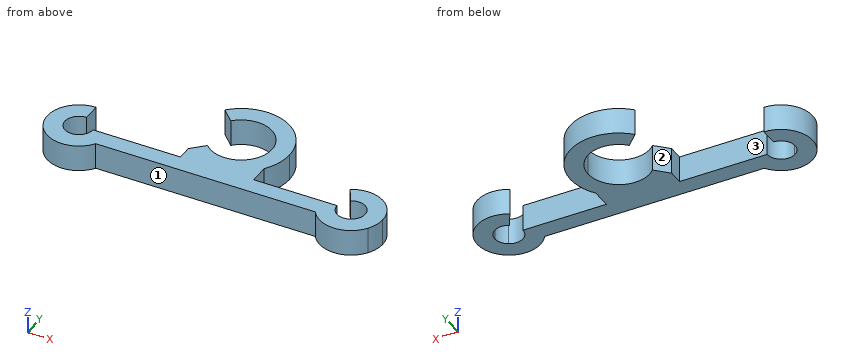
from build123d import *

# Parameters (mm, degrees)
F1_DEPTH = 3


with BuildPart() as f1:
    # F0 (on Top) → F1 (new body)
    with BuildSketch(Plane.XY):
        with BuildLine():
            Line((4.3997598665, -5.5), (0, -5.5))
            Line((0, -5.5), (-3.9389383459, -5.5))
            Line((-3.9389383459, -5.5), (-11.8838464236, -5.5))
            ThreePointArc((-11.8838464236, -5.5), (-12.0388519916, -6.5449944321), (-12.4905205142, -7.5))
            Line((-12.4905205142, -7.5), (12.4905205142, -7.5))
            ThreePointArc((12.4905205142, -7.5), (12.0388519916, -6.5449944321), (11.8838464236, -5.5))
            Line((11.8838464236, -5.5), (4.3997598665, -5.5))
        make_face()
        with BuildLine():
            ThreePointArc((-12.4905205142, -7.5), (-12.0388519916, -6.5449944321), (-11.8838464236, -5.5))
            Line((-11.8838464236, -5.5), (-13.8838464236, -5.5))
            ThreePointArc((-13.8838464236, -5.5), (-14.6838464236, -6.8856406461), (-16.2838464236, -6.8856406461))
            Line((-16.2838464236, -6.8856406461), (-16.638546962, -7.5))
            Line((-16.638546962, -7.5), (-12.4905205142, -7.5))
        make_face()
        with BuildLine():
            Line((-16.638546962, -7.5), (-16.2838464236, -6.8856406461))
            ThreePointArc((-16.2838464236, -6.8856406461), (-17.0293277457, -5.0858895278), (-15.4838464236, -3.9))
            Line((-15.4838464236, -3.9), (-15.4838464236, -1.9))
            ThreePointArc((-15.4838464236, -1.9), (-18.6587479969, -3.8029437252), (-18.4771723331, -7.5))
            Line((-18.4771723331, -7.5), (-16.638546962, -7.5))
        make_face()
        with BuildLine():
            Line((13.8838464236, -5.5), (11.8838464236, -5.5))
            ThreePointArc((11.8838464236, -5.5), (12.0388519916, -6.5449944321), (12.4905205142, -7.5))
            Line((12.4905205142, -7.5), (16.638546962, -7.5))
            Line((16.638546962, -7.5), (16.2838464236, -6.8856406461))
            ThreePointArc((16.2838464236, -6.8856406461), (14.6838464236, -6.8856406461), (13.8838464236, -5.5))
        make_face()
        with BuildLine():
            ThreePointArc((19.0838464236, -5.5), (17.2838464236, -2.3823085464), (13.6838464236, -2.3823085464))
            Line((13.6838464236, -2.3823085464), (14.6838464236, -4.1143593539))
            ThreePointArc((14.6838464236, -4.1143593539), (16.2838464236, -4.1143593539), (17.0838464236, -5.5))
            ThreePointArc((17.0838464236, -5.5), (16.8694870697, -6.3), (16.2838464236, -6.8856406461))
            Line((16.2838464236, -6.8856406461), (16.638546962, -7.5))
            Line((16.638546962, -7.5), (18.4771723331, -7.5))
            ThreePointArc((18.4771723331, -7.5), (18.9288408557, -6.5449944321), (19.0838464236, -5.5))
        make_face()
        with BuildLine():
            ThreePointArc((-2.5065971292, 2.4427383879), (1.3185048441, 3.2421512883), (3.5, 0))
            ThreePointArc((3.5, 0), (1.3185048441, -3.2421512883), (-2.5065971292, -2.4427383879))
            Line((-2.5065971292, -2.4427383879), (-3.9389383459, -3.8385888953))
            ThreePointArc((-3.9389383459, -3.8385888953), (-2.1374939855, -5.0676542366), (0, -5.5))
            ThreePointArc((0, -5.5), (2.4594957974, -4.9194390354), (4.3997598665, -3.3003201537))
            ThreePointArc((4.3997598665, -3.3003201537), (5.2176948582, -1.7394425449), (5.5, 0))
            ThreePointArc((5.5, 0), (2.0719361836, 5.0948091673), (-3.9389383459, 3.8385888953))
            Line((-3.9389383459, 3.8385888953), (-2.5065971292, 2.4427383879))
        make_face()
        with BuildLine():
            ThreePointArc((0, -5.5), (-2.1374939855, -5.0676542366), (-3.9389383459, -3.8385888953))
            Line((-3.9389383459, -3.8385888953), (-3.9389383459, -5.5))
            Line((-3.9389383459, -5.5), (0, -5.5))
        make_face()
        with BuildLine():
            ThreePointArc((4.3997598665, -3.3003201537), (2.4594957974, -4.9194390354), (0, -5.5))
            Line((0, -5.5), (4.3997598665, -5.5))
            Line((4.3997598665, -5.5), (4.3997598665, -3.3003201537))
        make_face()
        with BuildLine():
            Line((16.638546962, -7.5), (12.4905205142, -7.5))
            ThreePointArc((12.4905205142, -7.5), (15.4838464236, -9.1), (18.4771723331, -7.5))
            Line((18.4771723331, -7.5), (16.638546962, -7.5))
        make_face()
        with BuildLine():
            ThreePointArc((-18.4771723331, -7.5), (-15.4838464236, -9.1), (-12.4905205142, -7.5))
            Line((-12.4905205142, -7.5), (-16.638546962, -7.5))
            Line((-16.638546962, -7.5), (-18.4771723331, -7.5))
        make_face()
    extrude(amount=F1_DEPTH)


solid = f1.part
CAD build for the part. Positions are in the model's coordinates, mm. Face numbers are marked on the shaded views. A direction names the side the tool comes from. Coordinates: 2 decimals unless noted, no trailing zeros. Write each loop counter-clockwise with the first axis right and the second up, starting at its lowest first coordinate (ties: lowest second). Pieces come first, ordered by that corner, then holes. Notation, with made-up numbers: M -22.75,35 L 2.25,35 A21 ccw 2.25,49 Z; hole C -25,-27.5 d9. An arc over 180 degrees is marked long. Return JSON: item names as keys, results as strings.
Item 1: Drop flat-ended pins along their axis: pin 1 Ø1.5 at (x, z) = (-9.5, 1) entering from +Y; pin 2 Ø3 at (x, y) = (-5, -2.5) entering from +Z; pin 3 Ø0.9 at (x, z) = (3, 1.5) entering from -Y; pin 4 Ø1.1 at (y, z) = (-4.5, 1) entering from +X. Give the stop position or say it passes through.
Findings below:
{"pin 1": "stops at y = -5.5", "pin 2": "passes through", "pin 3": "stops at y = -7.5", "pin 4": "stops at x = 19.06"}
Item 2: Slice it at A-A, the plane y = -6.5. Write the cut outline in (x, z).
Findings below:
{"outline": "M -18.94,0 L -16.73,0 L -16.73,3 L -18.94,3 Z; M -14.23,0 L 14.23,0 L 14.23,3 L -14.23,3 Z; M 16.73,0 L 18.94,0 L 18.94,3 L 16.73,3 Z"}
Item 3: Slice it at C-C, the plane z = 2.1. Write the cut outline in (x, y), and give its area (3 significant figures).
Findings below:
{"outline": "M -15.48,-3.9 L -15.48,-1.9 A3.6 ccw long -12.49,-7.5 L 12.49,-7.5 A3.6 ccw long 13.68,-2.38 L 14.68,-4.11 A1.6 cw long 13.88,-5.5 L 4.4,-5.5 L 4.4,-3.3 A5.5 ccw -3.94,3.84 L -2.51,2.44 A3.5 cw long -2.51,-2.44 L -3.94,-3.84 L -3.94,-5.5 L -13.88,-5.5 A1.6 cw long Z", "area": "148 mm2"}
Item 4: Probe line 1 (X direction, y = -6.25, z = 2.8); line 2 (X direction, y = -6.5, z = 2.25); line 3 (Y direction, x = -12, z = 2.9). List the from-to ranges inside material, lowest first. Write a range as from..to.
Findings below:
{"line 1": "x = -19..-16.9, -14.07..14.07, 16.9..19", "line 2": "x = -18.94..-16.73, -14.23..14.23, 16.73..18.94", "line 3": "y = -7.5..-5.5"}
Item 5: Which spindle directions (+Z, -Z, +X, -X, +Y, -Y) get a long thin tool onto all of the face, cutting with end or side? Do the marked faces 1, 2 and 3. Say none if no direction does.
Findings below:
{"face 1": "+Z, -Z, -Y", "face 2": "+Z, -Z", "face 3": "+Z, -Z, +Y"}
Item 6: Slice it at D-D, the plane x = -7. Write the cut outline in (y, z).
Findings below:
{"outline": "M -7.5,0 L -5.5,0 L -5.5,3 L -7.5,3 Z"}
Item 7: Slice it at B-B, the plane x = 2. Write the cut outline in (y, z).
Findings below:
{"outline": "M -7.5,0 L -2.87,0 L -2.87,3 L -7.5,3 Z; M 2.87,0 L 5.12,0 L 5.12,3 L 2.87,3 Z"}
